Verification items for the finished model (mm, model axes). Face numbers are marked on the shaded views. Coordinates: 2 decimals unless noted, no trailing zeros. Order: outer loops, then holes, each group sorted by start corner. A loop starts at its lowest first (then second) coordinate and runs counter-clockwise, first axis right, second up. Notation, with made-up numbers: (69, -12.5) - (83, -12.5) arc R30 ccw to (83, 13.5) - close; hole circle Ø8 at (-29, 68). An arc over 180 degrees is marked (long way). Answer as CSV lines item,"result". Start each with the question number.
1. Mould release check, pull along X, two halves, no side actions. Record for the marked faces 1, 2 and 3: pulls with the +X half, pulls with the -X half, needs draft (parallel to the pull), parting line crosses it, or undercut.
2. Section check C-C (z = 8.5). Count the separate pieces of the cut face and the enclosed holes in it, and give its area (3 significant figures).
3. Section check B-B (x = 0). Record the cut outline in (y, z).
4. Material ranges on L1, parallel to X at y = 7, z = 6.75; L2, parallel to X at y = -8, z = 14.25; L3, parallel to Y at x = 113, z = 6.5, recorded low to high. Write a range as [from, to].
5. Go/stop test with flat-tipped pins: pin 1 (4 mm diameter, centred on x = 100.5, z = 4, fed in from -Y); pin 2 (1.5 mm diameter, centred on y = -2.5, z = 6, fed in from +X). Record where each tip stops, or that it passes through.
6. Section check A-A (y = -13.5). Record the cut outline in (x, z), and give its area (3 significant figures).
7. Section check D-D (x = 46). Record the cut outline in (y, z).
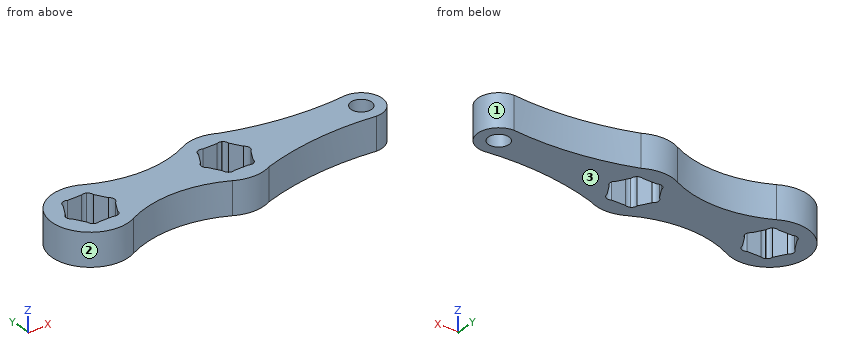
Autodesk Inventor part; units mm, degrees
ref_plane "YZ Plane" through (0, 0, 0) normal (1, 0, 0) x (0, 1, 0)
ref_plane "XZ Plane" through (0, 0, 0) normal (0, 1, 0) x (-1, 0, 0)
ref_plane "XY Plane" through (0, 0, 0) normal (0, 0, 1) x (1, 0, 0)
sketch "Sketch1" plane through (0, 0, 0) normal (0, 0, 1) x (1, 0, 0)
  line L0 (-11.4295, -0.0912) -> (-11.4381, -0.0912)
  line L1 (-5.798, 9.8601) -> (-5.7937, 9.8528)
  line L2 (5.6401, 9.9513) -> (5.6341, 9.9392)
  line L3 (11.4381, 0.0912) -> (11.4295, 0.0912)
  line L4 (5.798, -9.8601) -> (5.7937, -9.8528)
  line L5 (-5.6401, -9.9513) -> (-5.6341, -9.9392)
  arc A0 (-3.2667, 9.8803) -> (-7.0462, 7.6578) centre (-4.5062, 7.6633) ccw
  arc A1 (7.0443, 7.5633) -> (3.3664, 9.9332) centre (4.5062, 7.6633) ccw
  arc A2 (10.2075, -2.0801) -> (10.1371, 2.3037) centre (8.8895, 0.0912) ccw
  arc A3 (3.2667, -9.8803) -> (7.0462, -7.6578) centre (4.5062, -7.6633) ccw
  arc A4 (-7.0443, -7.5633) -> (-3.3664, -9.9332) centre (-4.5062, -7.6633) ccw
  arc A5 (-10.2075, 2.0801) -> (-10.1371, -2.3037) centre (-8.8895, -0.0912) ccw
  line L6 (-11.4295, -0.1058) -> (-11.4381, -0.0912)
  line L7 (-11.4381, -0.0912) -> (-11.4295, -0.076)
  line L8 (-10.2075, 2.0801) -> (-7.0462, 7.6578)
  line L9 (-5.8064, 9.8453) -> (-5.798, 9.8601)
  line L10 (-5.798, 9.8601) -> (-5.781, 9.8602)
  line L11 (5.6401, 9.9513) -> (5.6527, 9.9298)
  line L12 (-3.2667, 9.8803) -> (3.3664, 9.9332)
  line L13 (5.6098, 9.951) -> (5.6401, 9.9513)
  line L14 (7.0443, 7.5633) -> (10.1371, 2.3037)
  line L15 (11.4295, 0.1058) -> (11.4381, 0.0912)
  line L16 (11.4381, 0.0912) -> (11.4295, 0.076)
  line L17 (10.2075, -2.0801) -> (7.0462, -7.6578)
  line L18 (5.8064, -9.8453) -> (5.798, -9.8601)
  line L19 (5.798, -9.8601) -> (5.781, -9.8602)
  line L20 (-5.6401, -9.9513) -> (-5.6527, -9.9298)
  line L21 (-7.0443, -7.5633) -> (-10.1371, -2.3037)
  line L22 (3.2667, -9.8803) -> (-3.3664, -9.9332)
  line L23 (-5.6098, -9.951) -> (-5.6401, -9.9513)
  arc A6 (8.5907, 15.5669) -> (8.5907, -15.5669) centre (0, 0) ccw
  line L24 (52.0664, -0.0912) -> (52.0579, -0.0912)
  line L25 (57.6979, 9.8601) -> (57.7022, 9.8528)
  line L26 (69.136, 9.9513) -> (69.13, 9.9392)
  line L27 (74.9341, 0.0912) -> (74.9255, 0.0912)
  line L28 (69.294, -9.8601) -> (69.2897, -9.8528)
  line L29 (57.8559, -9.9513) -> (57.8619, -9.9392)
  arc A7 (60.2293, 9.8803) -> (56.4497, 7.6578) centre (58.9897, 7.6633) ccw
  arc A8 (70.5402, 7.5633) -> (66.8624, 9.9332) centre (68.0022, 7.6633) ccw
  arc A9 (73.7034, -2.0801) -> (73.633, 2.3037) centre (72.3855, 0.0912) ccw
  arc A10 (66.7626, -9.8803) -> (70.5422, -7.6578) centre (68.0022, -7.6633) ccw
  arc A11 (56.4517, -7.5633) -> (60.1296, -9.9332) centre (58.9897, -7.6633) ccw
  arc A12 (53.2885, 2.0801) -> (53.3589, -2.3037) centre (54.6064, -0.0912) ccw
  line L30 (52.0665, -0.1058) -> (52.0579, -0.0912)
  line L31 (52.0579, -0.0912) -> (52.0665, -0.076)
  line L32 (53.2885, 2.0801) -> (56.4497, 7.6578)
  line L33 (57.6895, 9.8453) -> (57.6979, 9.8601)
  line L34 (57.6979, 9.8601) -> (57.7149, 9.8602)
  line L35 (69.136, 9.9513) -> (69.1486, 9.9298)
  line L36 (60.2293, 9.8803) -> (66.8624, 9.9332)
  line L37 (69.1057, 9.951) -> (69.136, 9.9513)
  line L38 (70.5402, 7.5633) -> (73.633, 2.3037)
  line L39 (74.9255, 0.1058) -> (74.9341, 0.0912)
  line L40 (74.9341, 0.0912) -> (74.9254, 0.076)
  line L41 (73.7034, -2.0801) -> (70.5422, -7.6578)
  line L42 (69.3024, -9.8453) -> (69.294, -9.8601)
  line L43 (69.294, -9.8601) -> (69.277, -9.8602)
  line L44 (57.8559, -9.9513) -> (57.8433, -9.9298)
  line L45 (56.4517, -7.5633) -> (53.3589, -2.3037)
  line L46 (66.7626, -9.8803) -> (60.1296, -9.9332)
  line L47 (57.8862, -9.951) -> (57.8559, -9.9513)
  circle A13 centre (126.996, -0.1181) radius 4.7625
  arc A14 (124.9667, -9.5543) -> (125.0395, 9.3336) centre (126.996, -0.1181) ccw
  arc A15 (72.0866, 15.5669) -> (126.996, 9.5339) centre (113.0796, 135.7692) ccw
  arc A16 (126.996, -9.7701) -> (72.0866, -15.5669) centre (112.5559, -135.9465) ccw
  arc A17 (54.9053, -15.5669) -> (8.5907, -15.5669) centre (31.748, -60.7817) ccw
  arc A18 (8.5907, 15.5669) -> (54.9053, 15.5669) centre (31.748, 60.7817) ccw
  arc A19 (54.9053, -15.5669) -> (72.0866, -15.5669) centre (63.496, 0) ccw
  arc A20 (72.0866, 15.5669) -> (54.9053, 15.5669) centre (63.496, 0) ccw
  dimension "d19" = 9.525
  dimension "d21" = 19.304
  dimension "d22" = 127
  dimension "d23" = 127
  dimension "d24" = 50.8
  dimension "d25" = 50.8
extrude "Extrusion1" add sketch "Sketch1" along normal blind 15.24 contours A5 L6 L0 | L0 L7 A5 | L9 L1 A0 | L1 L10 A0 | A3 L4 L19 | A3 L18 L4 | L15 L3 A2 | A2 L3 L16 | A18 A20 A15 A14 A16 A19 A17 A6 | A12 L30 L24 | L24 L31 A12 | L33 L25 A7 | L25 L34 A7 | A10 L28 L43 | A10 L42 L28 | L39 L27 A9 | A9 L27 L40
properties part number "JB_CAD_FinalPt1"
Evaluation:
1,face 1,"pulls with the +X half"
1,face 2,"undercut"
1,face 3,"needs draft"
2,separate pieces,"1"
2,enclosed holes,"3"
2,area,"3,010 mm²"
3,outline,"(-17.78, 0) - (-9.91, 0) - (-9.91, 15.24) - (-17.78, 15.24) - close; (9.91, 0) - (17.78, 0) - (17.78, 15.24) - (9.91, 15.24) - close"
4,L1,"x = [-16.34, -7.42], [7.38, 56.08], [70.87, 133.51]"
4,L2,"x = [-15.88, -7.02], [7.02, 56.47], [70.52, 132.57]"
4,L3,"y = [-8.95, 8.77]"
5,pin 1,"stops at y = -9.73"
5,pin 2,"stops at x = 136.51"
6,outline,"(-11.57, 0) - (13.17, 0) - (13.17, 15.24) - (-11.57, 15.24) - close; (50.32, 0) - (78.85, 0) - (78.85, 15.24) - (50.32, 15.24) - close"
6,area,"812 mm²"
7,outline,"(-12.02, 0) - (12.02, 0) - (12.02, 15.24) - (-12.02, 15.24) - close"
